Part model, mm, in its own coordinate system. Face numbers are marked on the shaded views. Coordinates: 2 decimals unless noted, no trailing zeros. Order: outer loops, then holes, each group sorted by start corner. A loop starts at its lowest first (then second) coordinate and runs counter-clockwise, first axis right, second up.
1) Cut at B-B (z = 8). List the corners of the cut face in (x, y) (3 decimals), and give its area (3 significant figures).
2) Cut at A-A (x = -17.5). List the corners of the cut face in (y, z).
3) Cut at D-D (x = 4). List the corners of the cut face in (y, z).
4) Cut at C-C (y = 0). Give the number of separate pieces and of enclosed holes in the cut face, and give its area (3 significant figures).
5) Pin check, flat tips, straight feed: pin 1 Ø1.5 at (x, z) = (-24.5, 6) entering from -Y; pin 2 Ø5 at (x, y) = (6, -1.5) entering from +Z; pin 3 Ø4 at (y, z) = (-3.5, 7.5) entering from -X (3 decimals). Stop position of each tip, or through.
6) Wall check: L1, parallel to Y at x = 33.5, z = 8; L2, parallel to Y at x = -7.5, z = 2.2; L3, parallel to Z at x = -16, y = 1. Give the ranges that are in metal, low to high.
7) Mould opens along X. For the marked faces 1, 2, 3 and 4 say: +X half, -X half, draft (parallel to the pull), parting line (faces both ways), or undercut.
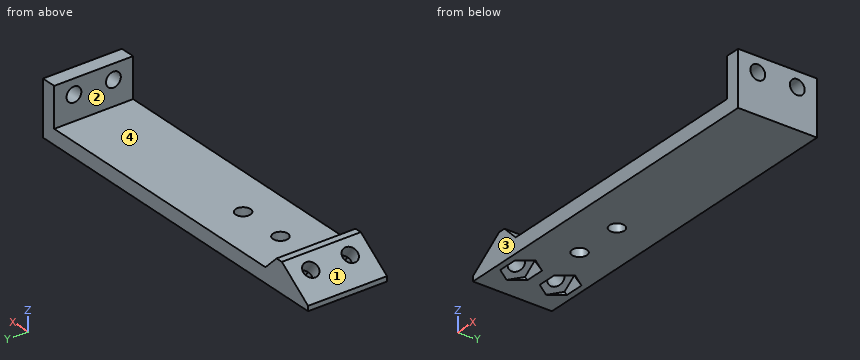
```python
from build123d import *

# Parameters (mm, degrees)
SKETCH1_W           = 70.85
SKETCH1_H           = 16
BOSS_EXTRUDE1_DEPTH = 3
SKETCH2_W           = 8.4
SKETCH2_H           = 16
BOSS_EXTRUDE2_DEPTH = 3
CHAMFER1_SIZE       = 5
CHAMFER1_SIZE2      = 7
SKETCH3_R           = 1.5
CUT_EXTRUDE1_DEPTH  = 3
CHAMFER2_SIZE       = 3
CUT_EXTRUDE2_START  = -3
CUT_EXTRUDE2_DEPTH  = 8
SKETCH5_W           = 3
SKETCH5_H           = 16
BOSS_EXTRUDE3_DEPTH = 8
SKETCH6_R           = 1.5
CUT_EXTRUDE3_DEPTH  = 8
SKETCH7_R           = 1.5
CUT_EXTRUDE4_DEPTH  = 10
SKETCH8_R           = 1.5
CUT_EXTRUDE5_DEPTH  = 10


with BuildPart() as part:
    # Sketch1 → Boss-Extrude1 (new body)
    with BuildSketch(Plane.XY):
        Rectangle(SKETCH1_W, SKETCH1_H)
    extrude(amount=BOSS_EXTRUDE1_DEPTH)

    # Sketch2 → Boss-Extrude2 (add)
    with BuildSketch(Plane.XY.offset(3)):
        with Locations((-31.225, 0)):
            Rectangle(SKETCH2_W, SKETCH2_H)
    extrude(amount=BOSS_EXTRUDE2_DEPTH)

    # Chamfer1
    chamfer1_edges = [part.edges().sort_by_distance(p)[0] for p in [
        (-35.425, 0, 6),
    ]]
    chamfer1_side = [part.faces().sort_by_distance(p)[0] for p in [
        (-35.425, 0, 3),
    ]]
    chamfer(chamfer1_edges, length=CHAMFER1_SIZE, length2=CHAMFER1_SIZE2, reference=chamfer1_side[0])

    # Sketch3 → Cut-Extrude1 (cut)
    with BuildSketch(Plane(origin=(-12.440878378, 0, 17.41722973), x_dir=(0.8137334712067354, 0, 0.5812381937190957), z_dir=(-0.5812381937190957, 0, 0.8137334712067354))):
        with Locations((-22.642944757, 4)):
            Circle(SKETCH3_R)
        with Locations((-22.642944757, -4)):
            Circle(SKETCH3_R)
    extrude(amount=-CUT_EXTRUDE1_DEPTH, mode=Mode.SUBTRACT)

    # Chamfer2
    chamfer2_edges = [part.edges().sort_by_distance(p)[0] for p in [
        (-27.025, 0, 3),
    ]]
    chamfer(chamfer2_edges, length=CHAMFER2_SIZE - 0.0001)  # a hair under: the kernel refuses the full size

    # Sketch4 → Cut-Extrude2 (cut)
    with BuildSketch(Plane(origin=(-12.440878378, 0, 17.41722973), x_dir=(0.8137334712067354, 0, 0.5812381937190959), z_dir=(-0.5812381937190958, 0, 0.8137334712067353)).offset(CUT_EXTRUDE2_START)):
        Polygon((-19.467518276, 4), (-21.055231516, 6.75), (-24.230657997, 6.75), (-25.818371237, 4), (-24.230657997, 1.25), (-21.055231516, 1.25), align=None)
        Polygon((-19.467518276, -4), (-21.055231516, -1.25), (-24.230657997, -1.25), (-25.818371237, -4), (-24.230657997, -6.75), (-21.055231516, -6.75), align=None)
    extrude(amount=-CUT_EXTRUDE2_DEPTH, mode=Mode.SUBTRACT)

    # Sketch5 → Boss-Extrude3 (add)
    with BuildSketch(Plane.XY.offset(3)):
        with Locations((33.925, 0)):
            Rectangle(SKETCH5_W, SKETCH5_H)
    extrude(amount=BOSS_EXTRUDE3_DEPTH)

    # Sketch6 → Cut-Extrude3 (cut)
    with BuildSketch(Plane(origin=(35.425, 0, 0), x_dir=(0, 0, -1), z_dir=(1, 0, 0))):
        with Locations((-8, 4)):
            Circle(SKETCH6_R)
        with Locations((-8, -4)):
            Circle(SKETCH6_R)
    extrude(amount=-CUT_EXTRUDE3_DEPTH, mode=Mode.SUBTRACT)

    # Sketch7 → Cut-Extrude4 (cut)
    with BuildSketch(Plane(origin=(0, 0, 0), x_dir=(-1, 0, 0), z_dir=(0, 0, -1))):
        with Locations((17.5, 0)):
            Circle(SKETCH7_R)
    extrude(amount=-CUT_EXTRUDE4_DEPTH, mode=Mode.SUBTRACT)

    # Sketch8 → Cut-Extrude5 (cut)
    with BuildSketch(Plane.XY.offset(3)):
        with Locations((-7.5, 0)):
            Circle(SKETCH8_R)
    extrude(amount=-CUT_EXTRUDE5_DEPTH, mode=Mode.SUBTRACT)


solid = part.part
```
Geometry check:
1. outline: (32.425, -8) - (35.425, -8) - (35.425, -5.5) - (32.425, -5.5) - close; (32.425, -2.5) - (35.425, -2.5) - (35.425, 2.5) - (32.425, 2.5) - close; (32.425, 5.5) - (35.425, 5.5) - (35.425, 8) - (32.425, 8) - close
1. area: 30.0 mm2
2. outline: (-8, 0) - (-1.5, 0) - (-1.5, 3) - (-8, 3) - close; (1.5, 0) - (8, 0) - (8, 3) - (1.5, 3) - close
3. outline: (-8, 0) - (8, 0) - (8, 3) - (-8, 3) - close
4. separate pieces: 3
4. enclosed holes: 0
4. area: 231 mm2
5. pin 1: passes through
5. pin 2: stops at z = 3
5. pin 3: stops at x = -29.125
6. L1: y = -8 to -5.5, -2.5 to 2.5, 5.5 to 8
6. L2: y = -8 to -1.5, 1.5 to 8
6. L3: z = 0 to 3
7. face 1: -X half
7. face 2: undercut
7. face 3: draft
7. face 4: undercut
